The listing builds one solid part. Answer for the finished solid, in the listing's coordinates (mm). Face numbers are marked on the shaded views. A direction names the side the tool comes from. Round coordinates to 2 decimals unless told otherwise and drop trailing zeros. Loops run counter-clockwise (first coordinate to the right, second up) from the corner with the lowest first, then second, coordinate; pieces in that order, holes last. Notation, with made-up numbers: M 53.5,51 L 84.5,51 A33 ccw 84.5,89 Z; hole C 61.25,83.25 d7. An arc over 180 degrees is marked long. Put each result on its own line as item: value. Start each with the question number.
(1) Section C-C, the plane x = -15 is taken. Determine the outline of the cut face in (y, z), then the cut area to 3 significant figures.
(2) Section B-B, the plane x = 0 is taken. Determine the outline of the cut face in (y, z), then the cut area to 3 significant figures.
(3) Straight lines are drawn through the part: line 1 (Y direction, x = 0, z = 14.5); line 2 (Z direction, x = 0, y = 52.5); line 3 (Y direction, x = 19, z = 6.5). For each, find the intervals that lie inside material, in ascending order.
(4) Section D-D, the plane z = 38 is taken. Determine the outline of the cut face in (x, y).
(5) Flat-ended cylindrical pins translate along their axes: P1, Ø12, axis at y = 85.5, z = 35, coming from the +X side; P2, Ø4, axis at y = -5.5, z = 17, coming from the -X side; P3, Ø5, axis at x = -30, z = 18.5, coming from the -Y side. Find the tip coordinate at first contact, or state that the pin passes through.
(6) Section A-A, the plane y = 0 is taken. Determine the outline of the cut face in (x, z), then the cut area to 3 significant figures.
(7) Which of the six approach directions +Z, -Z, +X, -X, +Y, -Y give full straight-line access (tool end or side, diameter ignored) to the marked faces 1, 2, 3 and 4?
(8) Determine the mould class of the marked faces 5, 6, 7 and 8 for opening direction Y: released by +Y, released by -Y, zero draft, split by the parting line, or undercut.
```python
from build123d import *

# Parameters (mm, degrees)
SKETCH1_R               = 22.5
BOSS_EXTRUDE1_DEPTH     = 50
CUT_EXTRUDE1_REACH      = 145.178
CUT_EXTRUDE1_END_RADIUS = 22.5
SKETCH3_R               = 10


with BuildPart() as part:
    # Sketch1 → Boss-Extrude1 (new body)
    with BuildSketch(Plane.XY):
        with BuildLine():
            Line((-25, 103.903355596), (-10, 91.316861128))
            Line((-10, 91.316861128), (10, 91.316861128))
            Line((10, 91.316861128), (25, 103.903355596))
            Line((25, 103.903355596), (35, 103.903355596))
            Line((35, 103.903355596), (35, 63.903355596))
            ThreePointArc((35, 63.903355596), (17.980602011, 51.434096177), (21.606705181, 30.649637701))
            ThreePointArc((21.606705181, 30.649637701), (0, -37.5), (-21.606705181, 30.649637701))
            ThreePointArc((-21.606705181, 30.649637701), (-17.980602011, 51.434096177), (-35, 63.903355596))
            Line((-35, 63.903355596), (-35, 103.903355596))
            Line((-35, 103.903355596), (-25, 103.903355596))
        make_face()
        Circle(SKETCH1_R, mode=Mode.SUBTRACT)
    extrude(amount=BOSS_EXTRUDE1_DEPTH)

    # Cut-Extrude1: up to this cylinder (the profile starts outside it)
    cut_extrude1_end = Plane(origin=(0, 0, 25), z_dir=(0, 0, -1)) * Cylinder(CUT_EXTRUDE1_END_RADIUS, 336.356, mode=Mode.PRIVATE)
    # Sketch3 → Cut-Extrude1 (cut, up to the surface)
    with BuildSketch(Plane(origin=(0, 91.316861128, 0), x_dir=(1, 0, 0), z_dir=(0, 1, 0)), mode=Mode.PRIVATE) as cut_extrude1_sk1:
        with Locations(Location((0, -25, 0), (0, 0, 270))):
            Circle(SKETCH3_R)
    cut_extrude1_tool1 = extrude(cut_extrude1_sk1.sketch, amount=-CUT_EXTRUDE1_REACH, mode=Mode.PRIVATE) - cut_extrude1_end
    add(cut_extrude1_tool1.solids().sort_by_distance((0, 91.316861, 25))[0], mode=Mode.SUBTRACT)


solid = part.part
```
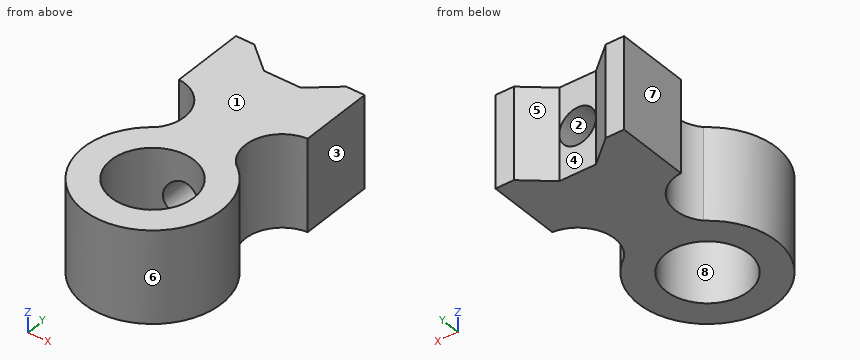
Recorded:
1. outline: M -34.37,0 L -16.77,0 L -16.77,50 L -34.37,50 Z; M 16.77,0 L 95.51,0 L 95.51,50 L 16.77,50 Z
1. area: 4,820 mm²
2. outline: M -37.5,0 L -22.5,0 L -22.5,50 L -37.5,50 Z; M 22.5,0 L 91.32,0 L 91.32,15 L 22.5,15 Z; M 22.5,35 L 91.32,35 L 91.32,50 L 22.5,50 Z
2. area: 2,810 mm²
3. line 1: y = -37.5 to -22.5, 22.5 to 91.32
3. line 2: z = 0 to 15, 35 to 50
3. line 3: y = -32.33 to -12.05, 12.05 to 34.34, 53.59 to 98.87
4. outline: M -35,63.9 A20 cw -21.61,30.65 A37.5 ccw long 21.61,30.65 A20 cw 35,63.9 L 35,103.9 L 25,103.9 L 10,91.32 L -10,91.32 L -25,103.9 L -35,103.9 Z; hole C 0,0 d45
5. P1: stops at x = 35
5. P2: stops at x = -37.34
5. P3: stops at y = -25.5
6. outline: M -37.5,0 L -22.5,0 L -22.5,50 L -37.5,50 Z; M 22.5,0 L 37.5,0 L 37.5,50 L 22.5,50 Z
6. area: 1,500 mm²
7. face 1: +Z, +X, -X, +Y, -Y
7. face 2: +Y
7. face 3: +Z, -Z, +X, +Y
7. face 4: +Z, -Z, +Y
8. face 5: released by +Y
8. face 6: undercut
8. face 7: zero draft
8. face 8: undercut
